Input: dimensioned drawing with shaded views. Units: mm. Origin: part minimum x, y, z. Round coordinates to 2 decimals unless told otherwise and drop trailing zeros. Loops run counter-clockwise (first coordinate to the right, second up) from the corner with the lowest first, then second, coordinate; pieces in that order, holes last. Notation, with made-up numbers: (16, 69) - (45, 69) arc R9 cw to (45, 80) - close; hole circle Ø8 at (65, -18). An arc over 180 degrees is marked (long way). One line per question, with ' | ' between items.
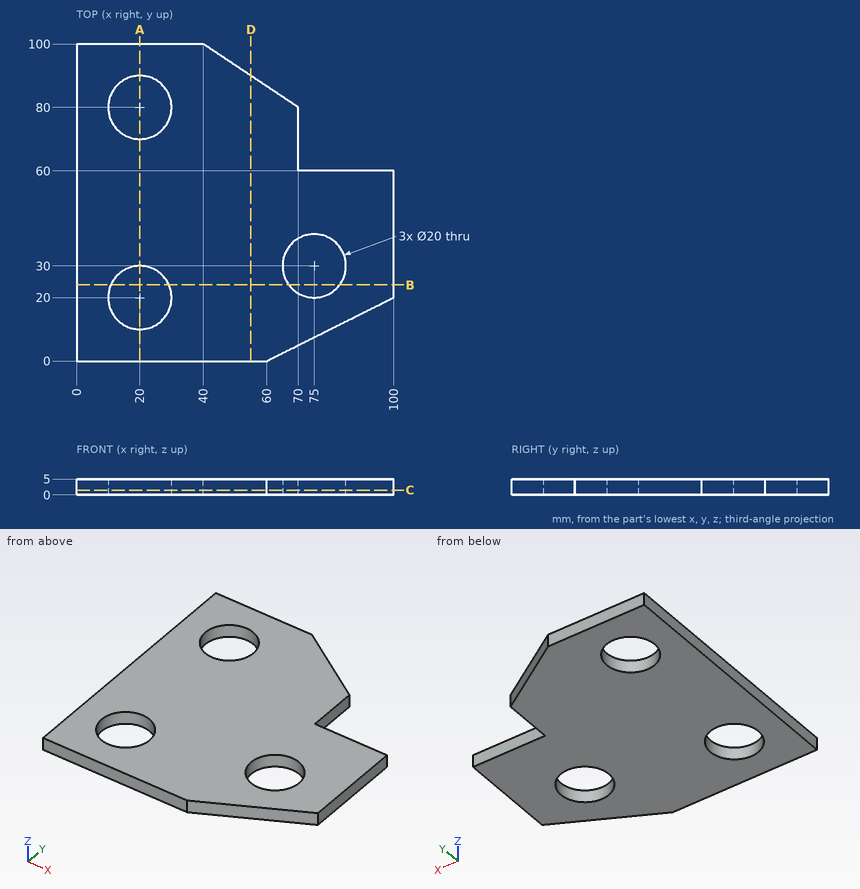
1. Material intervals for probe 1 along Y at (x, z) = (20, 1.75); probe 2 along X at (y, z) = (28, 1.45); probe 3 along X at (y, z) = (66, 0.45), sorted ascending.
Worked out:
probe 1: y = 0 to 10, 30 to 70, 90 to 100 | probe 2: x = 0 to 14, 26 to 65.2, 84.8 to 100 | probe 3: x = 0 to 70
2. Section query B-B, the plane y = 24. Return loops of the section in (x, z).
Worked out:
outline: (0, 0) - (10.83, 0) - (10.83, 5) - (0, 5) - close; (29.17, 0) - (67, 0) - (67, 5) - (29.17, 5) - close; (83, 0) - (100, 0) - (100, 5) - (83, 5) - close
3. Contact query for flat-ended pins moving along their axis: P1, Ø18, axis at x = 20, y = 20, coming from the +Z side; P2, Ø2.5, axis at x = 91, z = 1.5, coming from the +Y side; P3, Ø1, axis at y = 69, z = 3, coming from the +X side; P4, Ø3, axis at y = 12.5, z = 4, coming from the +X side. Output: stop coordinate, or through.
Worked out:
P1: passes through | P2: stops at y = 60 | P3: stops at x = 70 | P4: stops at x = 88
4. Section query D-D, the plane x = 55. Return loops of the section in (y, z).
Worked out:
outline: (0, 0) - (90, 0) - (90, 5) - (0, 5) - close
5. Section query C-C, the plane z = 1.45. Return loops of the section in (x, y).
Worked out:
outline: (0, 0) - (60, 0) - (100, 20) - (100, 60) - (70, 60) - (70, 80) - (40, 100) - (0, 100) - close; hole circle Ø20 at (20, 20); hole circle Ø20 at (20, 80); hole circle Ø20 at (75, 30)
6. Section query A-A, the plane x = 20. Return loops of the section in (y, z).
Worked out:
outline: (0, 0) - (10, 0) - (10, 5) - (0, 5) - close; (30, 0) - (70, 0) - (70, 5) - (30, 5) - close; (90, 0) - (100, 0) - (100, 5) - (90, 5) - close
